CAD build for the part. Positions are in the model's coordinates, mm. A direction names the side the tool comes from. Round coordinates to 2 decimals unless told otherwise and drop trailing zeros. Order: outer loops, then holes, each group sorted by start corner. A loop starts at its lowest first (then second) coordinate and runs counter-clockwise, first axis right, second up. Notation, with made-up numbers: (-33.5, 32.5) - (9.5, 32.5) arc R18 ccw to (9.5, 47.5) - close; hole circle Ø3 at (69, 16). An arc over 180 degrees is marked (long way). Write item = value, one per line.
from build123d import *

# Parameters (mm, degrees)
SKETCH1_R           = 11.5
SKETCH1_W           = 8
SKETCH1_H           = 8
BOSS_EXTRUDE1_DEPTH = 12
CUT_EXTRUDE1_DEPTH  = 12
CIRPATTERN1_COUNT   = 20


with BuildPart() as part:
    # Sketch1 → Boss-Extrude1 (new body)
    with BuildSketch(Plane.XY):
        Circle(SKETCH1_R)
        Rectangle(SKETCH1_W, SKETCH1_H, mode=Mode.SUBTRACT)
    extrude(amount=BOSS_EXTRUDE1_DEPTH)

    # Sketch2 → Cut-Extrude1 (cut)
    with BuildSketch(Plane.XY.offset(12)):
        with BuildLine():
            Line((0, 11.6), (1.5, 11.6))
            Line((1.5, 11.6), (0.8, 10.6))
            Line((0.8, 10.6), (0.559317479, 10))
            ThreePointArc((0.559317479, 10), (0, 9.642447684), (-0.559317479, 10))
            Line((-0.559317479, 10), (-0.8, 10.6))
            Line((-0.8, 10.6), (-1.5, 11.6))
            Line((-1.5, 11.6), (0, 11.6))
        make_face()
    cut_extrude1 = extrude(amount=-CUT_EXTRUDE1_DEPTH, mode=Mode.SUBTRACT)

    # CirPattern1: Cut-Extrude1 ×20 about axis
    cirpattern1_axis = Axis((0, 0, 0), (0, 0, 1))
    for i in range(1, CIRPATTERN1_COUNT):
        add(cut_extrude1.rotate(cirpattern1_axis, i * 360 / CIRPATTERN1_COUNT), mode=Mode.SUBTRACT)


solid = part.part
(1) Band-saw the part on B-B on y = 4.5. List the corners of the cut face in (x, z), plus the area to 3 significant figures.
Solved:
outline = (-10.18, 0) - (10.18, 0) - (10.18, 12) - (-10.18, 12) - close
area = 244 mm²
(2) Band-saw the part on A-A on x = -0.25. List the corners of the cut face in (y, z).
Solved:
outline = (-9.7, 0) - (-4, 0) - (-4, 12) - (-9.7, 12) - close; (4, 0) - (9.7, 0) - (9.7, 12) - (4, 12) - close
(3) Pull direction Y, two halves, no side cores. Call faces 4 (the cylindrical face through (-11.36, -1.79, 5.92)), 5 (the flat face through (-7.343, 8.266, 6.084)), 6 (the cylindrical face through (-7.795, 5.676, 6.084)): released by +Y, released by -Y, zero draft, split by the parting line, or undercut.
Solved:
face_4 = released by -Y
face_5 = released by +Y
face_6 = undercut
(4) Tool access for faces 1 (the flat face through (-11.015, 1.09, 6.084)), 2 (the flat face through (4, 0, 6)), 3 (the flat face through (1.09, 11.015, 6.084)): list every direction of +Z, -Z, +X, -X, +Y, -Y with a clear straight run to the whole face (end or side of a thin tool).
Solved:
face_1 = +Z, -Z, -X
face_2 = +Z, -Z
face_3 = +Z, -Z, +Y
(5) Drop flat-ended pins along their axis: pin 1 (4 mm diameter, centred on y = -2, z = 7, fed in from -X); pin 2 (3 mm diameter, centred on y = 5, z = 1.5, fed in from +X); pin 3 (2.5 mm diameter, centred on y = 0, z = 4, fed in from +X); pin 4 (4 mm diameter, centred on x = 7.5, z = 7, fed in from +Y). Give the stop position or say it passes through.
Solved:
pin_1 = -11.42
pin_2 = 10.43
pin_3 = 11.24
pin_4 = 10.1
(6) Probe line 1 along X through (y, z) = (-3.25, 9.75); line 2 along Y through (x, z) = (-9.25, 5.25); line 3 along Y through (x, z) = (-1, 1.5). List the from-to ranges inside material, lowest first.
Solved:
line_1 = -9.15 to -4, 4 to 9.15
line_2 = -5.59 to -3.52, -2.82 to 2.82, 3.52 to 5.59
line_3 = -10.89 to -4, 4 to 10.89
